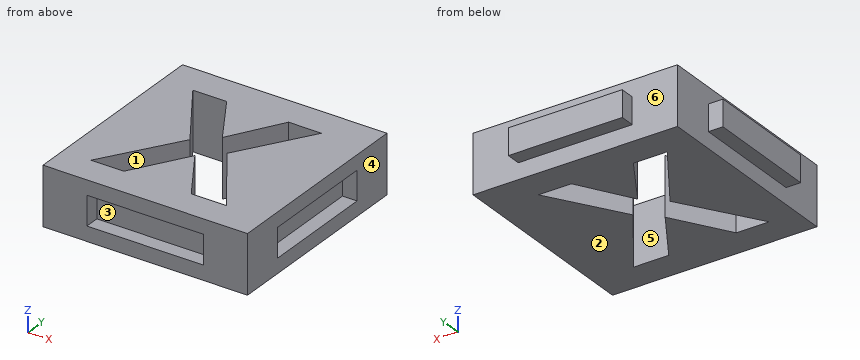
from build123d import *

# Parameters (mm, degrees)
F0_W     = 35.56
F0_H     = 35.56
F1_DEPTH = 5.08
F2_W     = 19.812
F2_H     = 4.572
F3_DEPTH = 2.54
F4_W     = 19.812
F4_H     = 4.572
F5_DEPTH = 2.54
F6_W     = 20.32
F6_H     = 5.08
F7_DEPTH = 2.54
F8_W     = 20.32
F8_H     = 5.08
F9_DEPTH = 2.54


with BuildPart() as f1:
    # F0 (on Top) → F1 (new body, symmetric)
    with BuildSketch(Plane.XY):
        Rectangle(F0_W, F0_H)
        Polygon((2.1111545139, -0.0055121528), (10.6219184028, -12.7), (4.5254774306, -12.7), (-1.3339409722, -3.175), (-7.1878472222, -12.7), (-12.9094618056, -12.7), (-4.5530381944, 0.2866319444), (-12.3747829861, 12.4850260417), (-6.4822916667, 12.4850260417), (-1.0583333333, 3.423046875), (4.26640625, 12.4850260417), (10.0155815972, 12.4850260417), align=None, mode=Mode.SUBTRACT)
    extrude(amount=F1_DEPTH, both=True)

    # F2 (on face) → F3 (join)
    with BuildSketch(Plane(origin=(0, 17.78, 0), x_dir=(-1, 0, 0), z_dir=(0, 1, 0))):
        Rectangle(F2_W, F2_H)
    extrude(amount=F3_DEPTH)

    # F4 (on face) → F5 (join)
    with BuildSketch(Plane(origin=(-17.78, 0, 0), x_dir=(0, -1, 0), z_dir=(-1, 0, 0))):
        Rectangle(F4_W, F4_H)
    extrude(amount=F5_DEPTH)

    # F6 (on face) → F7 (cut)
    with BuildSketch(Plane.XZ.offset(17.78)):
        Rectangle(F6_W, F6_H)
    extrude(amount=-F7_DEPTH, mode=Mode.SUBTRACT)

    # F8 (on face) → F9 (cut)
    with BuildSketch(Plane.YZ.offset(17.78)):
        Rectangle(F8_W, F8_H)
    extrude(amount=-F9_DEPTH, mode=Mode.SUBTRACT)


solid = f1.part
Input: part model. Units: mm. Frame: model coordinates. Face numbers are marked on the shaded views. A direction names the side the tool comes from. Give positions to 0.01 mm unless a question says otherwise; leave off trailing zeros. Loops run counter-clockwise (first coordinate to the right, second up) from the corner with the lowest first, then second, coordinate; pieces in that order, holes last. Notation, with made-up numbers: (76.25, 11) -> (90.25, 11) arc R31 ccw to (90.25, 47) -> close; hole circle Ø5 at (60, 82). An arc over 180 degrees is marked (long way). Answer as a JSON object with one key per item and string values. Group by question number.
Item 1: Cut plane B-B, the plane y = -4. Return the cut outline in (x, z), and give its area (3 significant figures).
Item 2: Cut plane C-C, the plane x = -2. Return the cut outline in (y, z).
Item 3: Line query: probe 1 along X at (y, z) = (-10.5, 2.5); probe 2 along Y at (x, z) = (15.5, -1); probe 3 along X at (y, z) = (-11.5, 1). Output: solid intervals per line, ascending.
Item 4: Pull-direction query (X, two-part tool) for the marked faces 4, 5 and 6; classes: released by +X, released by -X, zero draft, split by the parting line, or undercut.
Item 5: Pin query (flat end, axial travel): P1, Ø1, axis at y = 10, z = 3, coming from the -X side; P2, Ø2, axis at x = -19, y = 0.5, coming from the -Z side; P3, Ø4, axis at y = -4, z = -0.5, coming from the +X side. Return the tip coordinate at first contact, or that it passes through.
Item 6: Reachability of the marked faces 1, 2 and 3 from +Z, -Z, +X, -X, +Y, -Y: full face, straight path, thin tool, end or side. Return the list, or none.
Item 7: Cut plane D-D, the plane x = -9. Return the cut outline in (y, z).
Checks:
{
 "1": {"outline": "(-20.32, -2.29) -> (-17.78, -2.29) -> (-17.78, -5.08) -> (-7.31, -5.08) -> (-7.31, 5.08) -> (-17.78, 5.08) -> (-17.78, 2.29) -> (-20.32, 2.29) -> close; (-1.84, -5.08) -> (-0.83, -5.08) -> (-0.83, 5.08) -> (-1.84, 5.08) -> close; (4.79, -5.08) -> (17.78, -5.08) -> (17.78, -2.54) -> (15.24, -2.54) -> (15.24, 2.54) -> (17.78, 2.54) -> (17.78, 5.08) -> (4.79, 5.08) -> close", "area": "247 mm²"},
 "2": {"outline": "(-17.78, -5.08) -> (-4.26, -5.08) -> (-4.26, 5.08) -> (-17.78, 5.08) -> (-17.78, 2.54) -> (-15.24, 2.54) -> (-15.24, -2.54) -> (-17.78, -2.54) -> close; (5, -5.08) -> (17.78, -5.08) -> (17.78, -2.29) -> (20.32, -2.29) -> (20.32, 2.29) -> (17.78, 2.29) -> (17.78, 5.08) -> (5, 5.08) -> close"},
 "3": {"probe 1": "x = -17.78 to -11.49, -5.84 to 3.17, 9.15 to 17.78", "probe 2": "y = -17.78 to -10.16, 10.16 to 17.78", "probe 3": "x = -17.78 to -12.14, -6.45 to 3.79, 9.82 to 17.78"},
 "4": {"face 4": "released by +X", "face 5": "undercut", "face 6": "zero draft"},
 "5": {"P1": "stops at x = -17.78", "P2": "stops at z = -2.29", "P3": "stops at x = 15.24"},
 "6": {"face 1": "+Z, -Z", "face 2": "-Z, +X, -X, +Y, -Y", "face 3": "-Y"},
 "7": {"outline": "(-17.78, -5.08) -> (-12.7, -5.08) -> (-12.7, 5.08) -> (-17.78, 5.08) -> (-17.78, 2.54) -> (-15.24, 2.54) -> (-15.24, -2.54) -> (-17.78, -2.54) -> close; (-6.62, -5.08) -> (7.22, -5.08) -> (7.22, 5.08) -> (-6.62, 5.08) -> close; (12.49, -5.08) -> (17.78, -5.08) -> (17.78, -2.29) -> (20.32, -2.29) -> (20.32, 2.29) -> (17.78, 2.29) -> (17.78, 5.08) -> (12.49, 5.08) -> close"}
}
